from build123d import *

# Parameters (mm, degrees)
F1_DEPTH    = 75
F2_T2_ANGLE = 123.6693885688
F3_T2_ANGLE = 146.542163671
F4_T2_ANGLE = 137.6625417494
F5_T2_ANGLE = 106.0986339536


# Not quite as in the source:
# - a fillet or chamfer that OpenCascade refuses, or shapes differently, is made with other operations: its cross-section is extruded or revolved along the edge and cut away or added


with BuildPart() as f1:
    # F0 (on Front) → F1 (new body)
    with BuildSketch(Plane.XZ):
        with BuildLine():
            Line((0, 18.0245880038), (0, 8.2237206428))
            ThreePointArc((0, 8.2237206428), (21.1654297157, 6.8979891087), (42, 2.9415184316))
            ThreePointArc((42, 2.9415184316), (22.3131070658, 14.1395036835), (0, 18.0245880038))
        make_face()
        with BuildLine():
            ThreePointArc((-42, 2.9415184316), (-21.1654297157, 6.8979891087), (0, 8.2237206428))
            Line((0, 8.2237206428), (0, 18.0245880038))
            ThreePointArc((0, 18.0245880038), (-22.3131070658, 14.1395036835), (-42, 2.9415184316))
        make_face()
    extrude(amount=F1_DEPTH)

    # F2: chamfer of 10 on 1 edges, made by hand

    # F2_s1 → F2_t2 (revolve, cut)
    with BuildSketch(Plane(origin=(19.9711424115, 0, -37.3002397662), x_dir=(0, 1, 0), z_dir=(0.472017023, 0, -0.8815894339))):
        Polygon((-65, 43.3641317608), (-75, 33.3641317608), (-75, 43.3641317608), align=None)
    revolve(axis=Axis((0, -75, -47.9931074722), (0, -1, 0)), revolution_arc=F2_T2_ANGLE, mode=Mode.SUBTRACT)

    # F3: chamfer of 15 on 1 edges, made by hand

    # F3_s1 → F3_t2 (revolve, cut)
    with BuildSketch(Plane(origin=(13.2298564014, 0, -44.0166808787), x_dir=(0, 1, 0), z_dir=(0.2878439127, 0, -0.9576773371))):
        Polygon((-50, 52.2031716385), (-75.6066017178, 41.5965699207), (-65, 52.2031716385), align=None)
    revolve(axis=Axis((0, -65, -47.9931074722), (0, -1, 0)), revolution_arc=F3_T2_ANGLE, mode=Mode.SUBTRACT)

    # F4: chamfer of 13 on 1 edges, made by hand

    # F4_s1 → F4_t2 (revolve, cut)
    with BuildSketch(Plane(origin=(16.1615809903, 0, -41.7345888895), x_dir=(0, 1, 0), z_dir=(0.3611156728, 0, -0.9325210297))):
        Polygon((-37, 48.6866321803), (-62.0104339226, 43.7117475596), (-50, 48.6866321803), align=None)
    revolve(axis=Axis((0, -50, -47.9931074722), (0, -1, 0)), revolution_arc=F4_T2_ANGLE, mode=Mode.SUBTRACT)

    # F5: chamfer of 6 on 1 edges, made by hand

    # F5_s1 → F5_t2 (revolve, cut)
    with BuildSketch(Plane(origin=(23.0555472536, 0, -30.6506000272), x_dir=(0, 1, 0), z_dir=(0.6011273799, 0, -0.7991532226))):
        Polygon((-31, 37.1677245289), (-42.8847116824, 35.9971825968), (-37, 37.1677245289), align=None)
    revolve(axis=Axis((0, -37, -47.9931074722), (0, -1, 0)), revolution_arc=F5_T2_ANGLE, mode=Mode.SUBTRACT)


solid = f1.part
The model under review builds one solid part; all positions refer to its coordinate system, in mm. Coordinates: 2 decimals unless noted, no trailing zeros. Loops run counter-clockwise (first coordinate to the right, second up) from the corner with the lowest first, then second, coordinate; pieces in that order, holes last. Notation, with made-up numbers: (-20, 13) -> (22, 13) arc R30 cw to (22, 38) -> close; hole circle Ø2 at (47.5, 68.5). An arc over 180 degrees is marked (long way). Use a Markdown table: item, result. Add a question column.
1. Add section A-A on y = -19.5. Write out the cut boundary in (x, z), plus the area to 3 significant figures.
2. To check wall thickness, follow line 1 (Z direction, x = -15, y = -26); line 2 (Z direction, x = 5, y = -35.5); line 3 (X direction, y = -18, z = 11.25). State the ranges of each line that lie inside material, in increasing order.
3. Add section B-B on y = -32.5. Write out the cut boundary in (x, z).
4. Clearance check with flat-ended pins moving along their axes: pin 1 Ø4 at (y, z) = (-13.5, 8.5) entering from +X; pin 2 Ø2 at (x, z) = (-15, 15) entering from +Y; pin 3 Ø4 at (x, y) = (21, -47.5) entering from -Z; pin 4 Ø12 at (x, y) = (12.5, -21) entering from +Z. State where each tip first meets the part, or that it passes through.
Returned:
| question | item | result |
|---|---|---|
| 1 | outline | (-42, 2.94) arc R169.62 cw to (42, 2.94) arc R66.02 ccw to start |
| 1 | area | 569 mm² |
| 2 | line 1 | z = 7.56 to 16.3 |
| 2 | line 2 | z = 8.15 to 17.39 |
| 2 | line 3 | x = -29.13 to 29.13 |
| 3 | outline | (-41.66, 3.03) arc R169.62 cw to (41.66, 3.03) arc R65.87 ccw to start |
| 4 | pin 1 | stops at x = 37.27 |
| 4 | pin 2 | stops at y = 0 |
| 4 | pin 3 | stops at z = 6.66 |
| 4 | pin 4 | stops at z = 17.7 |
